The model under review builds one solid part; all positions refer to its coordinate system, in mm. Face numbers are marked on the shaded views. A direction names the side the tool comes from. Give positions to 0.01 mm unless a question says otherwise; leave off trailing zeros. Write each loop counter-clockwise with the first axis right and the second up, starting at its lowest first coordinate (ties: lowest second). Pieces come first, ordered by that corner, then holes.
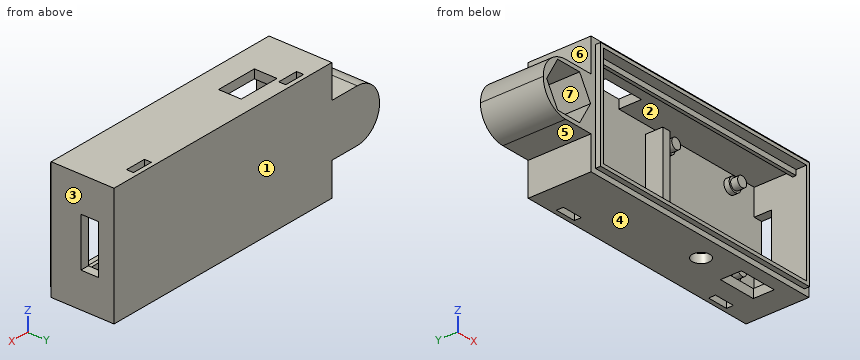
from build123d import *

# Parameters (mm, degrees)
SKETCH1_W             = 73
SKETCH1_H             = 34
BASE_DEPTH            = 4.5
SKETCH21_W            = 73
SKETCH21_H            = 34
EXTRUDE_UP_DEPTH      = 13.5
SKETCH22_W            = 68
SKETCH22_H            = 29
CUT_DOWN_DEPTH        = 13.5
SKETCH27_R            = 2
BOSS_EXTRUDE15_DEPTH  = 1.5
SKETCH29_R            = 2
BOSS_EXTRUDE16_DEPTH  = 1.5
SKETCH30_R            = 2
BOSS_EXTRUDE17_DEPTH  = 1.5
SKETCH28_R            = 2
BOSS_EXTRUDE18_DEPTH  = 1.5
SKETCH31_R            = 1.5
BOSS_EXTRUDE19_DEPTH  = 2
SKETCH32_R            = 1.5
BOSS_EXTRUDE20_DEPTH  = 2
SKETCH33_R            = 1.5
BOSS_EXTRUDE21_DEPTH  = 2
SKETCH34_R            = 1.5
BOSS_EXTRUDE22_DEPTH  = 2
SKETCH39_W            = 19
SKETCH39_H            = 1.3
WALL_SLIT_DEPTH       = 1.5
SKETCH41_W            = 2.5
SKETCH41_H            = 24
OUTSIDE_BLOCK_DEPTH   = 5
SKETCH44_W            = 2.5
SKETCH44_H            = 24
INSIDE_BLOCK_DEPTH    = 5
SKETCH45_W            = 12
SKETCH45_H            = 6.5
USB_HOLE_DEPTH        = 2.5
SKETCH62_W            = 70
SKETCH62_H            = 31
RAISE_LIP_DEPTH       = 1.5
SKETCH63_W            = 68
SKETCH63_H            = 29
CUT_LIP_DEPTH         = 1.5
SKETCH47_W            = 6
SKETCH47_H            = 2
TOP_TIE_HOLE_DEPTH    = 34
SKETCH48_W            = 6
SKETCH48_H            = 2
BOTTOM_TIE_HOLE_DEPTH = 34
SKETCH56_W            = 14
SKETCH56_H            = 5
WIRE_HOLE_DEPTH       = 2.5
SKETCH68_W            = 68
SKETCH68_H            = 1
RIGHT_LEDGE_DEPTH     = 1.5
SKETCH67_W            = 68
SKETCH67_H            = 1
LEFT_LEDGE_DEPTH      = 1.5
SKETCH65_W            = 16
SKETCH65_H            = 15
NUT_HOLE_SQUARE_DEPTH = 18
NUT_HOLE_FILLET_R     = 7.5
NUT_HOLE_HEX_DEPTH    = 15
SKETCH69_W            = 11
SKETCH69_H            = 6
CUT_EXTRUDE1_DEPTH    = 2.5
SKETCH70_R            = 2.5
CUT_EXTRUDE2_DEPTH    = 2.5


with BuildPart() as part:
    # Sketch1 → base (new body)
    with BuildSketch(Plane(origin=(0, 0, 0), x_dir=(1, 0, 0), z_dir=(0, 1, 0))):
        with Locations((5.291578947, 0.823157895)):
            Rectangle(SKETCH1_W, SKETCH1_H)
    extrude(amount=BASE_DEPTH)

    # Sketch21 → extrude up (add)
    with BuildSketch(Plane(origin=(0, 0, 0), x_dir=(-1, 0, 0), z_dir=(0, -1, 0))):
        with Locations((-5.291578947, 0.823157895)):
            Rectangle(SKETCH21_W, SKETCH21_H)
    extrude(amount=EXTRUDE_UP_DEPTH)

    # Sketch22 → cut down (cut)
    with BuildSketch(Plane(origin=(0, -13.5, 0), x_dir=(-1, 0, 0), z_dir=(0, -1, 0))):
        with Locations((-5.291578947, 0.823157895)):
            Rectangle(SKETCH22_W, SKETCH22_H)
    extrude(amount=-CUT_DOWN_DEPTH, mode=Mode.SUBTRACT)

    # Sketch27 → Boss-Extrude15 (add)
    with BuildSketch(Plane.XZ):
        with Locations(Location((31.141578947, -11.923157895, 0), (0, 0, 270))):
            Circle(SKETCH27_R)
    extrude(amount=BOSS_EXTRUDE15_DEPTH)

    # Sketch29 → Boss-Extrude16 (add)
    with BuildSketch(Plane.XZ):
        with Locations(Location((9.041578947, -11.923157895, 0), (0, 0, 270))):
            Circle(SKETCH29_R)
    extrude(amount=BOSS_EXTRUDE16_DEPTH)

    # Sketch30 → Boss-Extrude17 (add)
    with BuildSketch(Plane.XZ):
        with Locations(Location((9.041578947, 10.276842105, 0), (0, 0, 270))):
            Circle(SKETCH30_R)
    extrude(amount=BOSS_EXTRUDE17_DEPTH)

    # Sketch28 → Boss-Extrude18 (add)
    with BuildSketch(Plane.XZ):
        with Locations(Location((31.141578947, 10.276842105, 0), (0, 0, 270))):
            Circle(SKETCH28_R)
    extrude(amount=BOSS_EXTRUDE18_DEPTH)

    # Sketch31 → Boss-Extrude19 (add)
    with BuildSketch(Plane.XZ.offset(1.5)):
        with Locations(Location((31.141578947, -11.923157895, 0), (0, 0, 270))):
            Circle(SKETCH31_R)
    extrude(amount=BOSS_EXTRUDE19_DEPTH)

    # Sketch32 → Boss-Extrude20 (add)
    with BuildSketch(Plane.XZ.offset(1.5)):
        with Locations(Location((9.041578947, -11.923157895, 0), (0, 0, 270))):
            Circle(SKETCH32_R)
    extrude(amount=BOSS_EXTRUDE20_DEPTH)

    # Sketch33 → Boss-Extrude21 (add)
    with BuildSketch(Plane.XZ.offset(1.5)):
        with Locations(Location((9.041578947, 10.276842105, 0), (0, 0, 270))):
            Circle(SKETCH33_R)
    extrude(amount=BOSS_EXTRUDE21_DEPTH)

    # Sketch34 → Boss-Extrude22 (add)
    with BuildSketch(Plane.XZ.offset(1.5)):
        with Locations(Location((31.141578947, 10.276842105, 0), (0, 0, 270))):
            Circle(SKETCH34_R)
    extrude(amount=BOSS_EXTRUDE22_DEPTH)

    # Sketch39 → wall slit (cut)
    with BuildSketch(Plane.XY.offset(-15.323157895)):
        with Locations((-11.708421053, -4.85)):
            Rectangle(SKETCH39_W, SKETCH39_H)
    extrude(amount=-WALL_SLIT_DEPTH, mode=Mode.SUBTRACT)

    # Sketch41 → outside block (add)
    with BuildSketch(Plane.XZ):
        with Locations((-27.458421053, -0.823157895)):
            Rectangle(SKETCH41_W, SKETCH41_H)
    extrude(amount=OUTSIDE_BLOCK_DEPTH)

    # Sketch44 → inside block (add)
    with BuildSketch(Plane.XZ):
        with Locations((4.041578947, -0.823157895)):
            Rectangle(SKETCH44_W, SKETCH44_H)
    extrude(amount=INSIDE_BLOCK_DEPTH)

    # Sketch45 → usb hole (cut)
    with BuildSketch(Plane(origin=(0, 0, 13.676842105), x_dir=(-1, 0, 0), z_dir=(0, 0, -1))):
        with Locations((12.108421053, -3.25)):
            Rectangle(SKETCH45_W, SKETCH45_H)
    extrude(amount=-USB_HOLE_DEPTH, mode=Mode.SUBTRACT)

    # Sketch62 → raise lip (add)
    with BuildSketch(Plane.XZ.offset(13.5)):
        with Locations((5.291578947, -0.823157895)):
            Rectangle(SKETCH62_W, SKETCH62_H)
    extrude(amount=RAISE_LIP_DEPTH)

    # Sketch63 → cut lip (cut)
    with BuildSketch(Plane.XZ.offset(15)):
        with Locations((5.291578947, -0.823157895)):
            Rectangle(SKETCH63_W, SKETCH63_H)
    extrude(amount=-CUT_LIP_DEPTH, mode=Mode.SUBTRACT)

    # Sketch47 → top tie hole (cut)
    with BuildSketch(Plane.XY.offset(16.176842105)):
        with Locations((30.791578947, 2.25)):
            Rectangle(SKETCH47_W, SKETCH47_H)
    extrude(amount=-TOP_TIE_HOLE_DEPTH, mode=Mode.SUBTRACT)

    # Sketch48 → bottom tie hole (cut)
    with BuildSketch(Plane.XY.offset(16.176842105)):
        with Locations((-20.208421053, 2.25)):
            Rectangle(SKETCH48_W, SKETCH48_H)
    extrude(amount=-BOTTOM_TIE_HOLE_DEPTH, mode=Mode.SUBTRACT)

    # Sketch56 → wire hole (cut)
    with BuildSketch(Plane.ZY.offset(-39.291578947)):
        with Locations((-0.823157895, -2.5)):
            Rectangle(SKETCH56_W, SKETCH56_H)
    extrude(amount=-WIRE_HOLE_DEPTH, mode=Mode.SUBTRACT)

    # Sketch68 → right ledge (add)
    with BuildSketch(Plane.XY.offset(-15.323157895)):
        with Locations((5.291578947, -11.5)):
            Rectangle(SKETCH68_W, SKETCH68_H)
    extrude(amount=RIGHT_LEDGE_DEPTH)

    # Sketch67 → left ledge (add)
    with BuildSketch(Plane(origin=(0, 0, 13.676842105), x_dir=(-1, 0, 0), z_dir=(0, 0, -1))):
        with Locations((-5.291578947, -11.5)):
            Rectangle(SKETCH67_W, SKETCH67_H)
    extrude(amount=LEFT_LEDGE_DEPTH)

    # Sketch65 → nut hole square (add)
    with BuildSketch(Plane.XZ.offset(13.5)):
        with Locations((-39.208421053, -0.823157895)):
            Rectangle(SKETCH65_W, SKETCH65_H)
    extrude(amount=-NUT_HOLE_SQUARE_DEPTH)

    # nut hole fillet
    nut_hole_fillet_edges = [part.edges().sort_by_distance(p)[0] for p in [
        (-47.208421053, -4.5, -8.323157895),
        (-47.208421053, -4.5, 6.676842105),
    ]]
    fillet(nut_hole_fillet_edges, radius=NUT_HOLE_FILLET_R - 0.0001)  # a hair under: the kernel refuses the full size

    # Sketch66 → nut hole hex (cut)
    with BuildSketch(Plane.XZ.offset(13.5)):
        Polygon((-35.028097876, 5.551348835), (-42.388744229, 5.551348835), (-46.069067406, -0.823157895), (-42.388744229, -7.197664625), (-35.028097876, -7.197664625), (-31.347774699, -0.823157895), align=None)
    extrude(amount=-NUT_HOLE_HEX_DEPTH, mode=Mode.SUBTRACT)

    # Sketch69 → Cut-Extrude1 (cut)
    with BuildSketch(Plane.XY.offset(-15.323157895)):
        with Locations((28.791578947, -7)):
            Rectangle(SKETCH69_W, SKETCH69_H)
    extrude(amount=-CUT_EXTRUDE1_DEPTH, mode=Mode.SUBTRACT)

    # Sketch70 → Cut-Extrude2 (cut)
    with BuildSketch(Plane.XY.offset(-15.323157895)):
        with Locations((13.291578947, -7)):
            Circle(SKETCH70_R)
    extrude(amount=-CUT_EXTRUDE2_DEPTH, mode=Mode.SUBTRACT)


solid = part.part
1) Insertion check: pin 1 (0.8 mm diameter, centred on x = 4, z = 5, fed in from -Y); pin 2 (3.5 mm diameter, centred on x = -39, y = -9.5, fed in from -Z); pin 3 (17 mm diameter, centred on x = -6, z = 1.5, fed in from -Y). Each pin has a flat end and moves straight along its axis. Give the tip position at first contact, or say it passes through.
2) The part is to be moulded in two halves that separate along Y. For the marked faces 1, 2 and 3, say which applies: +Y half, -Y half, draft (parallel to the pull), parting line (faces both ways), or undercut.
3) Consider section C-C, the plane x = 2. Give the boundary of the cut face in (y, z), then the cut area to 4 significant figures.
4) Consider section A-A, the plane z = 2. State how many separate pieces and enclosed holes the cut face has, then the cut area to 3 significant figures.
5) Consider section B-B, the plane x = -15. Give the boundary of the cut face in (y, z), then the cut area to 3 significant figures.
6) Tool access review of the marked faces 4, 5, 6 and 7: name each direction out of +Z, -Z, +X, -X, +Y, -Y from which nothing blocks a thin tool from reaching the whole face with its end or side.
7) To check wall thickness, follow probe 1 along Z at (x, y) = (-27, -2); probe 2 along X at (y, z) = (-1.25, -9); probe 3 along Y at (x, z) = (31, -5). State the ranges of each line that lie inside material, in increasing order.
Answer block:
1. pin 1: stops at y = -5
1. pin 2: stops at z = -8.32
1. pin 3: stops at y = 0
2. face 1: +Y half
2. face 2: undercut
2. face 3: draft
3. outline: (-15, -16.32) - (-13.5, -16.32) - (-13.5, -17.82) - (4.5, -17.82) - (4.5, 16.18) - (-13.5, 16.18) - (-13.5, 14.68) - (-15, 14.68) - (-15, 13.68) - (-12, 13.68) - (-12, 12.18) - (-11, 12.18) - (-11, 13.68) - (0, 13.68) - (0, -15.32) - (-11, -15.32) - (-11, -13.82) - (-12, -13.82) - (-12, -15.32) - (-15, -15.32) - close
3. area: 226.5 mm2
4. separate pieces: 2
4. enclosed holes: 2
4. area: 494 mm2
5. outline: (-15, -16.32) - (-13.5, -16.32) - (-13.5, -17.82) - (4.5, -17.82) - (4.5, 16.18) - (0, 16.18) - (0, -15.32) - (-4.2, -15.32) - (-4.2, -16.82) - (-5.5, -16.82) - (-5.5, -15.32) - (-11, -15.32) - (-11, -13.82) - (-12, -13.82) - (-12, -15.32) - (-15, -15.32) - close; (-15, 13.68) - (-12, 13.68) - (-12, 12.18) - (-11, 12.18) - (-11, 13.68) - (-6.5, 13.68) - (-6.5, 16.18) - (-13.5, 16.18) - (-13.5, 14.68) - (-15, 14.68) - close
5. area: 208 mm2
6. face 4: -Z, +X, -X, +Y, -Y
6. face 5: -Z, -X, +Y, -Y
6. face 6: +Z, -X, +Y, -Y
6. face 7: -Y
7. probe 1: z = -17.82 to -15.32, -12.82 to 11.18, 13.68 to 16.18
7. probe 2: x = -31.21 to -26.21, 2.79 to 5.29, 39.29 to 41.79
7. probe 3: y = 0 to 1.25, 3.25 to 4.5
